Build history of the part. All positions in model axes, mm. Face numbers are marked on the shaded views. A direction names the side the tool comes from. Give positions to 0.01 mm unless a question says otherwise; leave off trailing zeros. Return JSON: item names as keys, results as strings. Group by question number.
Q1. Band-saw the part on A-A, the plane z = 1.1. Count the separate pieces of the cut face and the enclosed holes in it, then the cut area to 3 significant figures.
Q2. Tool access for the marked faces 1 and 2: list every direction of +Z, -Z, +X, -X, +Y, -Y with a clear straight run to the whole face (end or side of a thin tool).
Q3. Flat gauge pins, fed straight in: pin 1 Ø1 at (x, z) = (-22.5, 1) entering from -Y; pin 2 Ø2 at (y, z) = (-2.5, 0.5) entering from -X. Where does each tip first touch, or does it go through?
Q4. Wall check: probe 1 along Y at (x, z) = (11, 1.95); probe 2 along X at (y, z) = (0.75, 2.05); probe 3 along Y at (x, z) = (-11, 3.1). Give the ranges that are in metal, low to high.
Autodesk Fusion 360 part; units mm, degrees
sketch "Sketch1" plane through (0, 0, 0) normal (0, 0, 1) x (1, 0, 0)
  line L0 (-11, 0) -> (11, 0) construction
  circle A0 centre (-11, 0) radius 1.75
  circle A1 centre (-11, 0) radius 5
  circle A2 centre (11, 0) radius 1.75
  circle A3 centre (11, 0) radius 5
  line L1 (-11, 5) -> (11, 5)
  line L2 (11, -5) -> (-11, -5)
  dimension "d1" = 22
  dimension "d2" = 3.5
  dimension "d3" = 10
  dimension "d4" = 3.5
  dimension "d5" = 10
extrude "Extrude1" add sketch "Sketch1" along normal blind 4.5
sketch "Sketch2" plane through (0, 0, 4.5) normal (0, 0, 1) x (-1, 0, 0)
  circle A0 centre (-11, 0) radius 1.75
  circle A1 centre (11, 0) radius 1.75
  arc A2 (11, -5) -> (11, 5) centre (11, 0) ccw
  line L0 (11, 5) -> (-11, 5)
  arc A3 (-11, 5) -> (-11, -5) centre (-11, 0) ccw
  line L1 (-11, -5) -> (11, -5)
  line L2 (46.364, 12.87) -> (49.1808, 10.03)
  line L3 (49.1808, 10.03) -> (42.27, 6)
  line L4 (11, 0) -> (11, -5) construction
  spline S0 degree 5 poles (42.27, 6) (41.8597, 6.0483) (41.0377, 6.1242) (39.8004, 6.1754) (38.142, 6.1176) (36.0551, 5.832) (33.9568, 5.3324) (31.8528, 4.6259) (29.753, 3.7318) (27.6735, 2.6889) (25.6346, 1.5499) (23.6581, 0.3731) (21.7651, -0.7836) (19.9739, -1.8698) (18.2958, -2.85) (16.7347, -3.707) (15.5794, -4.2889) (14.7647, -4.667) (14.2444, -4.8933) (13.99, -5) knots 0 0 0 0 0 0 0.066667 0.133333 0.2 0.266667 0.333333 0.4 0.466667 0.533333 0.6 0.666667 0.733333 0.8 0.866667 0.933333 1 1 1 1 1 1
  line L5 (0, 0) -> (0, 5) construction
  spline S1 degree 5 poles (46.364, 12.87) (45.4848, 12.7904) (43.7223, 12.6243) (41.0656, 12.3544) (37.4975, 11.9526) (32.991, 11.3756) (28.4344, 10.7175) (23.8239, 9.9723) (19.158, 9.1377) (14.4396, 8.2182) (9.6729, 7.2207) (5.8243, 6.3656) (2.9193, 5.6943) (0.9744, 5.2336) (0, 5) knots 0 0 0 0 0 0 0.1 0.2 0.3 0.4 0.5 0.6 0.7 0.8 0.9 1 1 1 1 1 1
  line L6 (11, 0) -> (11, 5) construction
  line L7 (0, 5) -> (11, 5)
  line L8 (13.99, -5) -> (11, -5)
  point P0 (31.52, 4.45)
  point P1 (20.61, -1.48)
  point P2 (24.52, 10.07)
  dimension "d10" = 4
  dimension "d11" = 8
  dimension "d12" = 31.27
  dimension "d13" = 11
  dimension "d14" = 15.03
  dimension "d15" = 17.87
  dimension "d16" = 9.45
  dimension "d17" = 3.52
  dimension "d18" = 2.99
  dimension "d19" = 9.61
  dimension "d20" = 20.52
  dimension "d21" = 13.52
  dimension "d22" = 15.07
extrude "Extrude2" add sketch "Sketch2" against normal up to surface (4.5 mm away) contours A2 L0 L2 L3 S0 S1 L7 L8
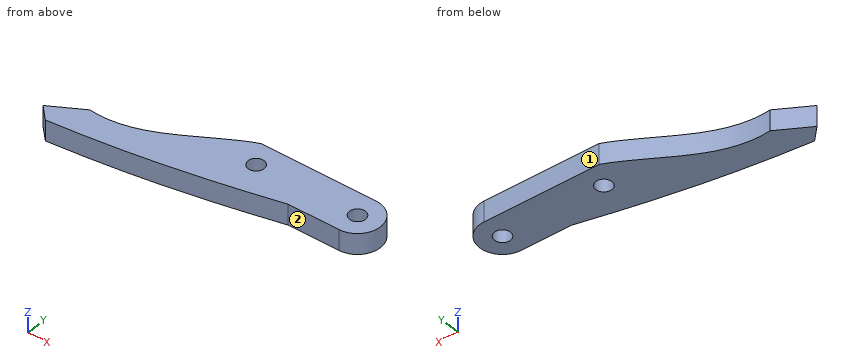
From the geometry:
{
 "1": {"separate pieces": "1", "enclosed holes": "2", "area": "561 mm^2"},
 "2": {"face 1": "+Z, -Z, +X, -X, +Y", "face 2": "+Z, -Z, +X, -Y"},
 "3": {"pin 1": "stops at y = -9.81", "pin 2": "stops at x = -29.34"},
 "4": {"probe 1": "y = -5 to -1.75, 1.75 to 5", "probe 2": "x = -21.82 to -12.58, -9.42 to 9.42, 12.58 to 15.94", "probe 3": "y = -7.49 to -1.75, 1.75 to 5"}
}
